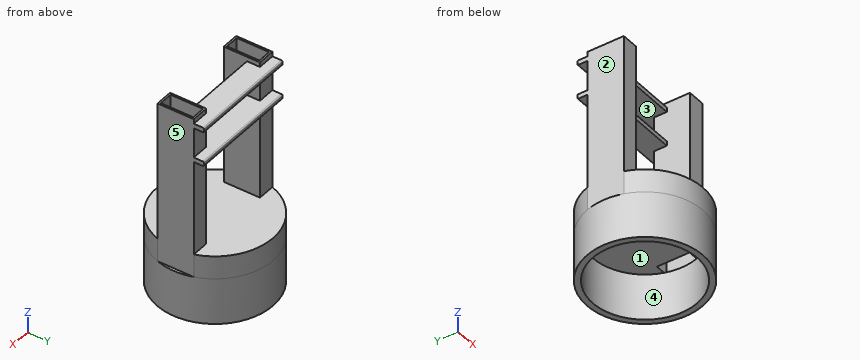
from build123d import *

# Parameters (mm, degrees)
IZIM1_W                      = 75
IZIM1_H                      = 156.12494996
Y_KSEKLIK_EKSTR_ZYON2_DEPTH  = 100
IZIM3_W                      = 75
IZIM3_H                      = 156.12494996
Y_KSEKLIK_EKSTR_ZYON3_DEPTH  = 600
Y_KSEKLIK_EKSTR_ZYON9_DEPTH  = 475
IZIM12_W                     = 59
IZIM12_H                     = 140.12494996
KES_EKSTR_ZYON3_DEPTH        = 781.324451751
Y_KSEKLIK_EKSTR_ZYON10_START = 200
IZIM13_R                     = 250
Y_KSEKLIK_EKSTR_ZYON10_DEPTH = 200
IZIM15_R                     = 225
KES_EKSTR_ZYON5_DEPTH        = 200


with BuildPart() as part:
    # Çizim1 → Yükseklik-Ekstrüzyon2 (new body)
    with BuildSketch(Plane.XY):
        with BuildLine():
            Line((162.5, 78.06247498), (237.5, 78.06247498))
            ThreePointArc((237.5, 78.06247498), (0, 250), (-237.5, 78.06247498))
            Line((-237.5, 78.06247498), (-162.5, 78.06247498))
            Line((-162.5, 78.06247498), (-162.5, -78.06247498))
            Line((-162.5, -78.06247498), (-237.5, -78.06247498))
            ThreePointArc((-237.5, -78.06247498), (0, -250), (237.5, -78.06247498))
            Line((237.5, -78.06247498), (162.5, -78.06247498))
            Line((162.5, -78.06247498), (162.5, 78.06247498))
        make_face()
        with Locations((-200, 0)):
            Rectangle(IZIM1_W, IZIM1_H)
        with Locations((200, 0)):
            Rectangle(IZIM1_W, IZIM1_H)
    extrude(amount=Y_KSEKLIK_EKSTR_ZYON2_DEPTH)

    # Çizim3 → Yükseklik-Ekstrüzyon3 (add)
    with BuildSketch(Plane.XY.offset(100)):
        with Locations((200, 0)):
            Rectangle(IZIM3_W, IZIM3_H)
        with Locations((-200, 0)):
            Rectangle(IZIM3_W, IZIM3_H)
    extrude(amount=Y_KSEKLIK_EKSTR_ZYON3_DEPTH)

    # Çizim5 → Yükseklik-Ekstrüzyon9 (add, through all)
    with BuildSketch(Plane.ZY.offset(237.5)):
        with BuildLine():
            Line((680, 22.081308318), (660, 22.081308318))
            Line((660, 22.081308318), (660, 117.081308318))
            ThreePointArc((660, 117.081308318), (661.464466094, 120.616842224), (665, 122.081308318))
            Line((665, 122.081308318), (675, 122.081308318))
            ThreePointArc((675, 122.081308318), (678.535533906, 120.616842224), (680, 117.081308318))
            Line((680, 117.081308318), (680, 22.081308318))
        make_face()
        with BuildLine():
            Line((530, 22.081308318), (510, 22.081308318))
            Line((510, 22.081308318), (510, 117.081308318))
            ThreePointArc((510, 117.081308318), (511.464466094, 120.616842224), (515, 122.081308318))
            Line((515, 122.081308318), (525, 122.081308318))
            ThreePointArc((525, 122.081308318), (528.535533906, 120.616842224), (530, 117.081308318))
            Line((530, 117.081308318), (530, 22.081308318))
        make_face()
    extrude(amount=-Y_KSEKLIK_EKSTR_ZYON9_DEPTH)

    # Çizim12 → Kes-Ekstrüzyon3 (cut, through all)
    with BuildSketch(Plane.XY.offset(700)):
        with Locations((-200, 0)):
            Rectangle(IZIM12_W, IZIM12_H)
        with Locations((200, 0)):
            Rectangle(IZIM12_W, IZIM12_H)
    extrude(amount=-KES_EKSTR_ZYON3_DEPTH, mode=Mode.SUBTRACT)

    # Çizim13 → Yükseklik-Ekstrüzyon10 (add)
    with BuildSketch(Plane(origin=(0, 0, 0), x_dir=(-1, 0, 0), z_dir=(0, 0, -1)).offset(Y_KSEKLIK_EKSTR_ZYON10_START)):
        Circle(IZIM13_R)
    extrude(amount=-Y_KSEKLIK_EKSTR_ZYON10_DEPTH)

    # Çizim15 → Kes-Ekstrüzyon5 (cut)
    with BuildSketch(Plane(origin=(0, 0, -200), x_dir=(-1, 0, 0), z_dir=(0, 0, -1))):
        Circle(IZIM15_R)
    extrude(amount=-KES_EKSTR_ZYON5_DEPTH, mode=Mode.SUBTRACT)


solid = part.part
The listing builds one solid part. Answer for the finished solid, in the listing's coordinates (mm). Face numbers are marked on the shaded views. A direction names the side the tool comes from. Give positions to 0.01 mm unless a question says otherwise; leave off trailing zeros. Write each loop counter-clockwise with the first axis right and the second up, starting at its lowest first coordinate (ties: lowest second). Pieces come first, ordered by that corner, then holes.
1) Section D-D (z = 58.5) is taken. Write down the section's boundary in (x, y), and give its area (3 significant figures).
2) Given P1, Ø4, axis at y = 52.5, z = 88, coming from the +X side; P2, Ø8, axis at x = 52, z = 669.5, coming from the +Y side; P3, Ø10, axis at x = 93, y = -136, coming from the +Z side; P4, Ø4.5, axis at x = 220.5, y = 22, coming from the +Z side, each flat-ended and moving along its own axis, determine where each tip first touches the part or whether it passes through.
3) A tool of negligible diameter and unlimited length cuts with its end or side. For the marked faces 4 and 5, from which of +Z, -Z, +X, -X, +Y, -Y can it reach the whole face along a straight path? Write none if from no direction.
4) Section A-A (z = 559.5) is taken. Write down the section's boundary in (x, y), and give its area (3 significant figures).
5) Find the intervals of material crossed by L1, parallel to Z at x = 211, y = 80.5; L2, parallel to Z at x = -16, y = 92; L3, parallel to X at y = 3, z = 470.5, in increasing order.
6) For a pull along Z with two mould halves and no side action, classify the marked faces 1, 2 and 3 as pulls with the +Z half, pulls with the -Z half, needs draft (parallel to the pull), parting line crosses it, or undercut.
7) Section C-C (x = 0) is taken. Write down the section's boundary in (y, z), and give its area (3 significant figures).
8) Section B-B (y = 0) is taken. Write down the section's boundary in (x, z), and give its area (3 significant figures).
Response:
1. outline: (-237.5, -78.06) arc R250 ccw to (237.5, -78.06) - (237.5, 78.06) arc R250 ccw to (-237.5, 78.06) - close; hole (-229.5, -70.06) - (-170.5, -70.06) - (-170.5, 70.06) - (-229.5, 70.06) - close; hole (170.5, -70.06) - (229.5, -70.06) - (229.5, 70.06) - (170.5, 70.06) - close
1. area: 177,000 mm2
2. P1: stops at x = 237.5
2. P2: stops at y = 122.08
2. P3: stops at z = 100
2. P4: passes through
3. face 4: -Z
3. face 5: +Z, +X, +Y, -Y
4. outline: (-237.5, -78.06) - (-162.5, -78.06) - (-162.5, 78.06) - (-237.5, 78.06) - close; (162.5, -78.06) - (237.5, -78.06) - (237.5, 78.06) - (162.5, 78.06) - close; hole (-229.5, -70.06) - (-170.5, -70.06) - (-170.5, 70.06) - (-229.5, 70.06) - close; hole (170.5, -70.06) - (229.5, -70.06) - (229.5, 70.06) - (170.5, 70.06) - close
4. area: 6,880 mm2
5. L1: z = -200 to 100, 510 to 530, 660 to 680
5. L2: z = 0 to 100, 510 to 530, 660 to 680
5. L3: x = -237.5 to -229.5, -170.5 to -162.5, 162.5 to 170.5, 229.5 to 237.5
6. face 1: pulls with the -Z half
6. face 2: needs draft
6. face 3: undercut
7. outline: (-250, -200) - (-225, -200) - (-225, 0) - (225, 0) - (225, -200) - (250, -200) - (250, 100) - (-250, 100) - close; (22.08, 510) - (117.08, 510) arc R5 ccw to (122.08, 515) - (122.08, 525) arc R5 ccw to (117.08, 530) - (22.08, 530) - close; (22.08, 660) - (117.08, 660) arc R5 ccw to (122.08, 665) - (122.08, 675) arc R5 ccw to (117.08, 680) - (22.08, 680) - close
7. area: 64,000 mm2
8. outline: (-250, -200) - (-225, -200) - (-225, 0) - (-229.5, 0) - (-229.5, 700) - (-237.5, 700) - (-237.5, 0) - (-250, 0) - close; (-170.5, 0) - (170.5, 0) - (170.5, 700) - (162.5, 700) - (162.5, 100) - (-162.5, 100) - (-162.5, 700) - (-170.5, 700) - close; (225, -200) - (250, -200) - (250, 0) - (237.5, 0) - (237.5, 700) - (229.5, 700) - (229.5, 0) - (225, 0) - close
8. area: 64,900 mm2
